Could you check a few things on this model? Use its own coordinates, in mm. Face numbers are marked on the shaded views. Round coordinates to 2 decimals unless told otherwise and drop trailing zeros. Return JSON: item names as keys, results as strings.
from build123d import *

# Parameters (mm, degrees)
SKETCH1_W                             = 90
SKETCH1_H                             = 95
BOSS_EXTRUDE1_DEPTH                   = 102.2
SKETCH2_R                             = 29.25
CUT_EXTRUDE1_DEPTH                    = 1
SKETCH3_R                             = 27.25
BOSS_EXTRUDE2_DEPTH                   = 1
TAP_DRILL_FOR_M4_TAP1_D               = 3.3
TAP_DRILL_FOR_M4_TAP1_DEPTH           = 5
TAP_DRILL_FOR_M4_TAP1_CSINK_D         = 3.35
TAP_DRILL_FOR_M4_TAP1_CSINK_ANGLE     = 90
TAP_DRILL_FOR_M4_TAP1_TIP             = 0.991420021
TAP_DRILL_FOR_M4_TAP2_D               = 3.3
TAP_DRILL_FOR_M4_TAP2_DEPTH           = 5
TAP_DRILL_FOR_M4_TAP2_CSINK_D         = 3.35
TAP_DRILL_FOR_M4_TAP2_CSINK_ANGLE     = 90
TAP_DRILL_FOR_M4_TAP2_TIP             = 0.991420021
TAP_DRILL_FOR_1_4_20_TAP1_D           = 5.1054
TAP_DRILL_FOR_1_4_20_TAP1_DEPTH       = 5
TAP_DRILL_FOR_1_4_20_TAP1_CSINK_D     = 6.3754
TAP_DRILL_FOR_1_4_20_TAP1_CSINK_ANGLE = 90
TAP_DRILL_FOR_1_4_20_TAP1_TIP         = 1.533816902
FILLET1_R                             = 5
CHAMFER1_SIZE                         = 1
SKETCH13_R                            = 12.7
CUT_EXTRUDE2_DEPTH                    = 1


with BuildPart() as part:
    # Sketch1 → Boss-Extrude1 (new body)
    with BuildSketch(Plane.XY):
        Rectangle(SKETCH1_W, SKETCH1_H)
    extrude(amount=-BOSS_EXTRUDE1_DEPTH)

    # Sketch2 → Cut-Extrude1 (cut)
    with BuildSketch(Plane.XY):
        with Locations((0, 2.5)):
            Circle(SKETCH2_R)
    extrude(amount=-CUT_EXTRUDE1_DEPTH, mode=Mode.SUBTRACT)

    # Sketch3 → Boss-Extrude2 (add)
    with BuildSketch(Plane.XY.offset(-1)):
        with Locations((0, 2.5)):
            Circle(SKETCH3_R)
    extrude(amount=BOSS_EXTRUDE2_DEPTH)

    # Tap Drill for M4 Tap1
    with Locations(Plane.XY):
        with Locations((-40, 42.5), (40, 42.5), (-40, -42.5), (40, -42.5)):
            CounterSinkHole(TAP_DRILL_FOR_M4_TAP1_D / 2, TAP_DRILL_FOR_M4_TAP1_CSINK_D / 2, depth=TAP_DRILL_FOR_M4_TAP1_DEPTH, counter_sink_angle=TAP_DRILL_FOR_M4_TAP1_CSINK_ANGLE)
            with Locations((0, 0, -(TAP_DRILL_FOR_M4_TAP1_DEPTH + TAP_DRILL_FOR_M4_TAP1_TIP / 2))):  # 118° drill point
                Cone(0, TAP_DRILL_FOR_M4_TAP1_D / 2, TAP_DRILL_FOR_M4_TAP1_TIP, mode=Mode.SUBTRACT)

    # Tap Drill for M4 Tap2
    with Locations(Plane(origin=(0, -47.5, 0), x_dir=(-1, 0, 0), z_dir=(0, -1, 0))):
        with Locations((-30, 83.9), (30, 83.9)):
            CounterSinkHole(TAP_DRILL_FOR_M4_TAP2_D / 2, TAP_DRILL_FOR_M4_TAP2_CSINK_D / 2, depth=TAP_DRILL_FOR_M4_TAP2_DEPTH, counter_sink_angle=TAP_DRILL_FOR_M4_TAP2_CSINK_ANGLE)
            with Locations((0, 0, -(TAP_DRILL_FOR_M4_TAP2_DEPTH + TAP_DRILL_FOR_M4_TAP2_TIP / 2))):  # 118° drill point
                Cone(0, TAP_DRILL_FOR_M4_TAP2_D / 2, TAP_DRILL_FOR_M4_TAP2_TIP, mode=Mode.SUBTRACT)

    # Tap Drill for 1/4-20 Tap1
    with Locations(Plane(origin=(0, -47.5, 0), x_dir=(-1, 0, 0), z_dir=(0, -1, 0))):
        with Locations((0, 48.9)):
            CounterSinkHole(TAP_DRILL_FOR_1_4_20_TAP1_D / 2, TAP_DRILL_FOR_1_4_20_TAP1_CSINK_D / 2, depth=TAP_DRILL_FOR_1_4_20_TAP1_DEPTH, counter_sink_angle=TAP_DRILL_FOR_1_4_20_TAP1_CSINK_ANGLE)
            with Locations((0, 0, -(TAP_DRILL_FOR_1_4_20_TAP1_DEPTH + TAP_DRILL_FOR_1_4_20_TAP1_TIP / 2))):  # 118° drill point
                Cone(0, TAP_DRILL_FOR_1_4_20_TAP1_D / 2, TAP_DRILL_FOR_1_4_20_TAP1_TIP, mode=Mode.SUBTRACT)

    # Fillet1
    fillet1_edges = [part.edges().sort_by_distance(p)[0] for p in [
        (45, -47.5, -51.1),
        (-45, -47.5, -51.1),
        (-45, 47.5, -51.1),
        (45, 47.5, -51.1),
    ]]
    fillet(fillet1_edges, radius=FILLET1_R)

    # Chamfer1
    chamfer1_edges = [part.edges().sort_by_distance(p)[0] for p in [
        (0, -47.5, 0),
        (0, -47.5, -102.2),
        (45, 0, 0),
        (0, 47.5, 0),
        (-45, 0, 0),
        (43.535533906, 46.035533906, 0),
        (-43.535533906, 46.035533906, 0),
        (-43.535533906, -46.035533906, 0),
        (43.535533906, -46.035533906, 0),
        (45, 0, -102.2),
        (-45, 0, -102.2),
        (0, 47.5, -102.2),
        (43.535533906, 46.035533906, -102.2),
        (-43.535533906, 46.035533906, -102.2),
        (-43.535533906, -46.035533906, -102.2),
        (43.535533906, -46.035533906, -102.2),
    ]]
    chamfer(chamfer1_edges, length=CHAMFER1_SIZE)

    # Sketch13 → Cut-Extrude2 (cut)
    with BuildSketch(Plane.XY):
        with Locations((0, 2.5)):
            Circle(SKETCH13_R)
    extrude(amount=-CUT_EXTRUDE2_DEPTH, mode=Mode.SUBTRACT)


solid = part.part
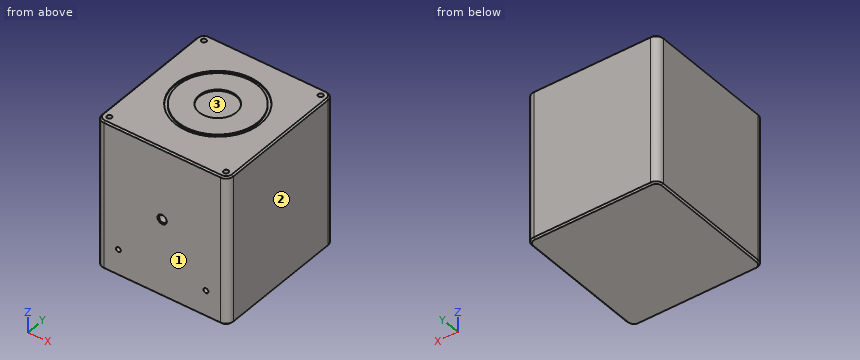
1) Will these pins go through, and if not, where does the flat tip stop? pin 1 Ø3 at (x, y) = (-4, 2.5) entering from +Z; pin 2 Ø3 at (x, y) = (-40, 42.5) entering from +Z; pin 3 Ø6 at (x, z) = (0, -48.9) entering from -Y.
Return value:
{"pin 1": "z = -1", "pin 2": "z = -5.09", "pin 3": "y = -47.31"}
2) Thinking about a two-plate mould opening in Y: for the marked faces 1, 2 and 3, which applies, pulls with the +Y half, pulls with the -Y half, needs draft (parallel to the pull), parting line crosses it, or undercut?
Return value:
{"face 1": "pulls with the -Y half", "face 2": "needs draft", "face 3": "undercut"}
3) If I drill on probe 1 along X at (y, z) = (-42.5, -1.1); probe 2 along Y at (x, z) = (40, -2); probe 3 along Z at (x, y) = (-30, -43), over which ranges is the centre line in solid material (lowest first)? Write a range as [from, to].
Return value:
{"probe 1": "[-45, -41.65], [-38.35, 38.35], [41.65, 45]", "probe 2": "[-47.5, -44.15], [-40.85, 40.85], [44.15, 47.5]", "probe 3": "[-102.2, -85.55], [-82.25, 0]"}
